The drawing under review shows one solid part. Ordinate dimensions are in mm from its lowest x, y, z. Round coordinates to 2 decimals unless told otherwise and drop trailing zeros. Order: outer loops, then holes, each group sorted by start corner. A loop starts at its lowest first (then second) coordinate and runs counter-clockwise, first axis right, second up. Notation, with made-up numbers: (-5, -19.75) -> (38, -19.75) arc R30 cw to (38, 19.25) -> close; hole circle Ø11 at (33, 13.25). An arc over 180 degrees is marked (long way). Use a Markdown table: item, result. Add a question column.
1) Consider section C-C (z = 741.5). State the section outline as (x, y) points (3 decimals), plus the area to 3 significant figures.
2) Clearance check with flat-ended pins moving along their axes: P1, Ø15, axis at x = 27, z = 245.5, coming from the -Y side (3 decimals); P2, Ø3, axis at x = 26, y = 3, coming from the -Z side; P3, Ø5, axis at x = 28.5, y = 2.5, coming from the +Z side; P4, Ø6, axis at y = 7, z = 470.5, coming from the -X side. State where each tip first meets the part, or that it passes through.
3) Wall thickness on line 1 along Z through (x, y) = (28.5, 8.5); line 2 along Y through (x, z) = (37, 486) (3 decimals): over which ranges is each line inside the solid? List them lowest first. Write a range as [from, to].
4) Consider section B-B (x = 15). State the section outline as (y, z) points (3 decimals).
5) Consider section A-A (y = 5.75). State the section outline as (x, z) points.
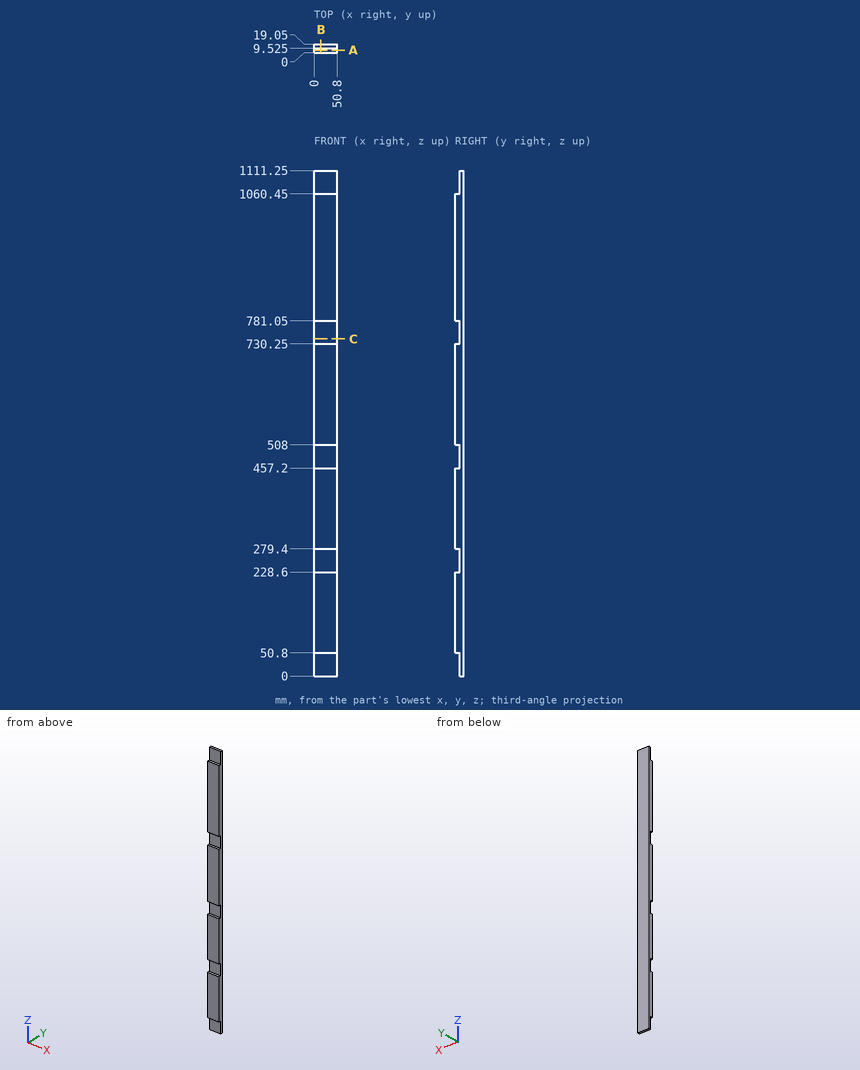
Results list:
| question | item | result |
|---|---|---|
| 1 | outline | (0, 9.525) -> (50.8, 9.525) -> (50.8, 19.05) -> (0, 19.05) -> close |
| 1 | area | 484 mm2 |
| 2 | P1 | y = 9.525 |
| 2 | P2 | z = 50.8 |
| 2 | P3 | z = 1060.45 |
| 2 | P4 | x = 0 |
| 3 | line 1 | [50.8, 228.6], [279.4, 457.2], [508, 730.25], [781.05, 1060.45] |
| 3 | line 2 | [9.525, 19.05] |
| 4 | outline | (0, 50.8) -> (9.525, 50.8) -> (9.525, 0) -> (19.05, 0) -> (19.05, 1111.25) -> (9.525, 1111.25) -> (9.525, 1060.45) -> (0, 1060.45) -> (0, 781.05) -> (9.525, 781.05) -> (9.525, 730.25) -> (0, 730.25) -> (0, 508) -> (9.525, 508) -> (9.525, 457.2) -> (0, 457.2) -> (0, 279.4) -> (9.525, 279.4) -> (9.525, 228.6) -> (0, 228.6) -> close |
| 5 | outline | (0, 50.8) -> (50.8, 50.8) -> (50.8, 228.6) -> (0, 228.6) -> close; (0, 279.4) -> (50.8, 279.4) -> (50.8, 457.2) -> (0, 457.2) -> close; (0, 508) -> (50.8, 508) -> (50.8, 730.25) -> (0, 730.25) -> close; (0, 781.05) -> (50.8, 781.05) -> (50.8, 1060.45) -> (0, 1060.45) -> close |
